Source: CAD feature listing. Evaluate the final solid. Frame: model axes, mm. A direction names the side the tool comes from. Round coordinates to 2 decimals unless told otherwise and drop trailing zeros. Order: outer loops, then holes, each group sorted by start corner. A loop starts at its lowest first (then second) coordinate and runs counter-clockwise, first axis right, second up. Notation, with made-up numbers: M -6,50.5 L 29,50.5 A10 ccw 29,65.5 Z; hole C 1,2.25 d4. An arc over 180 degrees is marked long. Answer as CSV lines item,"result". Start each with the question number.
Item 1: Set-up query: faces 1 (the face through (21, 38.289, 22)), 2 (the face through (-35.93, 41.36, -3.13)), 3 (the face through (-3.841, 13, 22)). Return all of +Z, -Z, +X, -X, +Y, -Y with unobstructed straight access to the full face (end or side cutting, diameter ignored); none if empty.
Item 2: Section query B-B on y = 36. Return the cut outline in (x, z).
Item 3: Section query C-C on z = 22. Return the cut outline in (x, y), plus the area to 3 significant figures.
Item 4: Line query: line 1 (X direction, y = 32, z = -2.5); line 2 (Z direction, x = -20.5, y = 13); line 3 (Y direction, x = 24, z = 15.5). Output: solid intervals per line, ascending. Write a range as [from, to].
Item 5: Section query A-A on z = -13. Return the cut outline in (x, y).
Item 6: Section query D-D on x = 44.5. Return the cut outline in (y, z).
Item 7: First-contact query: P1, Ø14.5, axis at x = 46.96, y = 31.94, coming from the +Z side; P2, Ø6, axis at y = 20, z = 2.5, coming from the +X side; P3, Ø8, axis at y = 36.5, z = -9, coming from the +X side. Flat tips, straight axial feed; report the tip coordinate or a pass-through.
Item 8: Pull-direction query (Y, two-part tool) for faces 4 (the face through (-67.335, 32.498, -9.392)), 5 (the face through (-3.841, 51, 22)), 6 (the face through (52.825, 29.507, -12.611)); classes: +Y half, -Y half, draft (parallel to the pull), parting line (faces both ways), or undercut.
from build123d import *

# Parameters (mm, degrees)
F1_DEPTH  = 19.05
F2_R      = 11.176
F3_DEPTH  = 6.35
F4_R      = 6.35
F5_DEPTH  = 19.051
F6_R      = 25.4
F7_DEPTH  = 31.75
F8_R      = 14.351
F9_DEPTH  = 50.801
F11_DEPTH = 19.05
F13_DEPTH = 19.05


with BuildPart() as f1:
    # F0 (on Top) → F1 (new body)
    with BuildSketch(Plane.XY):
        with BuildLine():
            ThreePointArc((-41.940726, 57.339477), (-23.980214, 49.899989), (-16.540726, 31.939477))
            ThreePointArc((-16.540726, 31.939477), (-23.980214, 13.978964), (-41.940726, 6.539477))
            Line((-41.940726, 6.539477), (46.959274, 6.539477))
            ThreePointArc((46.959274, 6.539477), (21.559274, 31.939477), (46.959274, 57.339477))
            Line((46.959274, 57.339477), (-41.940726, 57.339477))
        make_face()
        with BuildLine():
            ThreePointArc((-41.940726, 6.539477), (-23.980214, 13.978964), (-16.540726, 31.939477))
            ThreePointArc((-16.540726, 31.939477), (-23.980214, 49.899989), (-41.940726, 57.339477))
            ThreePointArc((-41.940726, 57.339477), (-67.340726, 31.939477), (-41.940726, 6.539477))
        make_face()
        with BuildLine():
            ThreePointArc((72.359274, 31.939477), (64.919786, 49.899989), (46.959274, 57.339477))
            ThreePointArc((46.959274, 57.339477), (21.559274, 31.939477), (46.959274, 6.539477))
            ThreePointArc((46.959274, 6.539477), (64.919786, 13.978964), (72.359274, 31.939477))
        make_face()
    extrude(amount=-F1_DEPTH)

    # F2 (on face) → F3 (cut)
    with BuildSketch(Plane.XY):
        with Locations((-41.940726, 31.939477)):
            Circle(F2_R)
        with Locations((46.959274, 31.939477)):
            Circle(F2_R)
    extrude(amount=-F3_DEPTH, mode=Mode.SUBTRACT)

    # F4 (on face) → F5 (cut, through all)
    with BuildSketch(Plane.XY):
        with Locations((-41.940726, 31.939477)):
            Circle(F4_R)
        with Locations((46.959274, 31.939477)):
            Circle(F4_R)
    extrude(amount=-F5_DEPTH, mode=Mode.SUBTRACT)

    # F6 (on face) → F7 (join)
    with BuildSketch(Plane.XY):
        with Locations((2.509274, 31.939477)):
            Circle(F6_R)
    extrude(amount=F7_DEPTH)

    # F8 (on face) → F9 (cut, through all)
    with BuildSketch(Plane.XY.offset(31.75)):
        with Locations((2.509274, 31.939477)):
            Circle(F8_R)
    extrude(amount=-F9_DEPTH, mode=Mode.SUBTRACT)

    # F10 (on face) → F11 (cut)
    with BuildSketch(Plane.XY.offset(31.75)):
        Polygon((8.859274, 57.339477), (2.509274, 57.339477), (-3.840726, 57.339477), (-3.840726, 6.539477), (8.859274, 6.539477), align=None)
    extrude(amount=-F11_DEPTH, mode=Mode.SUBTRACT)

    # F12 (on face) → F13 (cut)
    with BuildSketch(Plane.XY.offset(31.75)):
        Polygon((27.909274, 25.589477), (27.909274, 31.939477), (27.909274, 38.289477), (-22.890726, 38.289477), (-22.890726, 25.589477), align=None)
    extrude(amount=-F13_DEPTH, mode=Mode.SUBTRACT)


solid = f1.part
Results:
1,face 1,"+Z, +X, -X"
1,face 2,"+Z"
1,face 3,"+Z, +Y, -Y"
2,outline,"M -67.01,-19.05 L -46.82,-19.05 L -46.82,-6.35 L -52.35,-6.35 L -52.35,0 L -67.01,0 Z; M -37.06,-19.05 L -11.26,-19.05 L -11.26,12.7 L -22.56,12.7 L -22.56,0 L -31.53,0 L -31.53,-6.35 L -37.06,-6.35 Z; M 16.27,-19.05 L 42.08,-19.05 L 42.08,-6.35 L 36.55,-6.35 L 36.55,0 L 27.58,0 L 27.58,12.7 L 16.27,12.7 Z; M 51.84,-19.05 L 72.03,-19.05 L 72.03,0 L 57.37,0 L 57.37,-6.35 L 51.84,-6.35 Z"
3,outline,"M -22.08,25.59 A25.4 ccw -3.84,7.35 L -3.84,19.07 A14.35 cw -10.36,25.59 Z; M -22.08,38.29 L -10.36,38.29 A14.35 cw -3.84,44.81 L -3.84,56.53 A25.4 ccw Z; M 8.86,7.35 A25.4 ccw 27.1,25.59 L 15.38,25.59 A14.35 cw 8.86,19.07 Z; M 8.86,44.81 A14.35 cw 15.38,38.29 L 27.1,38.29 A25.4 ccw 8.86,56.53 Z"
3,area,"808 mm^2"
4,line 1,"[-67.34, -53.12], [-30.76, -11.84], [16.86, 35.78], [58.14, 72.36]"
4,line 2,"[-19.05, 0]"
4,line 3,"[18.4, 25.59], [38.29, 45.48]"
5,outline,"M -41.94,6.54 L 46.96,6.54 A25.4 ccw 72.36,31.94 A25.4 ccw 46.96,57.34 L -41.94,57.34 A25.4 ccw Z; hole C -41.94,31.94 d12.7; hole C 2.51,31.94 d28.7; hole C 46.96,31.94 d12.7"
6,outline,"M 6.54,-19.05 L 26.09,-19.05 L 26.09,-6.35 L 21.04,-6.35 L 21.04,0 L 6.54,0 Z; M 37.79,-19.05 L 57.34,-19.05 L 57.34,0 L 42.84,0 L 42.84,-6.35 L 37.79,-6.35 Z"
7,P1,"z = -6.35"
7,P2,"x = 70.19"
7,P3,"x = 72.35"
8,face 4,"parting line"
8,face 5,"draft"
8,face 6,"undercut"
